```python
from build123d import *

# Parameters (mm, degrees)
F0_W     = 64.9276450276
F0_H     = 21.2974622846
F0_W_2   = 4.8806965351
F0_H_2   = 10.0571289659
F1_DEPTH = 25.4
F2_DEPTH = 25.4


with BuildPart() as f1:
    # F0 (on Right) → F1 (new body)
    with BuildSketch(Plane.YZ):
        Polygon((42.2991216183, -21.2974622846), (42.2991216183, 21.2974622846), (4.8806965351, 21.2974622846), (0, 21.2974622846), (-42.2991216183, 21.2974622846), (-42.2991216183, 0), (-42.2991216183, -21.2974622846), align=None)
        with Locations((-74.7629441321, 10.6487311423)):
            Rectangle(F0_W, F0_H)
        with Locations((2.4403482676, 26.3260267675)):
            Rectangle(F0_W_2, F0_H_2)
    extrude(amount=F1_DEPTH)

    # F2 (add): a face of the model
    f2_faces = [f1.faces().sort_by_distance(p)[0] for p in [
        (0, -20.5074649501, 3.1809669358),
    ]]
    extrude(f2_faces, amount=F2_DEPTH)


solid = f1.part
```
Here's how the part is built. I have some questions about the finished solid (model axes, mm). A direction names the side the tool comes from. Coordinates: 2 decimals unless noted, no trailing zeros. Order: outer loops, then holes, each group sorted by start corner. A loop starts at its lowest first (then second) coordinate and runs counter-clockwise, first axis right, second up.
1) Imagine slicing it at C-C on z = -17.5. List the corners of the cut face in (x, y) for me, and give its area (3 significant figures).
2) Will these pins go through, and if not, where does the flat tip stop? pin 1 (5 mm diameter, centred on x = 2.5, y = 23.5, fed in from +Z); pin 2 (17 mm diameter, centred on x = -8, z = -9.5, fed in from -Y); pin 3 (8 mm diameter, centred on x = -6.5, z = 28.5, fed in from +Y).
3) Which directions (+Z, -Z, +X, -X, +Y, -Y) give clear straight access to the entire face, cutting with the end or side of a thin tool? Please do faces 1 (the face through (0, -42.299, -10)), 2 (the face through (0, 24, 21.297)), 3 (the face through (0, 0, 26)).
4) Imagine slicing it at B-B on y = -57. List the corners of the cut face in (x, z) for me.
5) Imagine slicing it at A-A on x = -5. List the corners of the cut face in (y, z) for me.
6) I need wall thicknesses on line 1 (Y direction, x = 5.5, z = -5.5); line 2 (Z direction, x = 15, y = -81); line 3 (Y direction, x = 12.5, z = 29). Which ranges of each line are inside material? Lowest first, please.
Response values:
1. outline: (-25.4, -42.3) - (25.4, -42.3) - (25.4, 42.3) - (-25.4, 42.3) - close
1. area: 4,300 mm2
2. pin 1: stops at z = 21.3
2. pin 2: stops at y = -42.3
2. pin 3: stops at y = 4.88
3. face 1: -Z, +X, -X, -Y
3. face 2: +Z, +X, -X, +Y
3. face 3: +Z, +X, -X, -Y
4. outline: (-25.4, 0) - (25.4, 0) - (25.4, 21.3) - (-25.4, 21.3) - close
5. outline: (-107.23, 0) - (-42.3, 0) - (-42.3, -21.3) - (42.3, -21.3) - (42.3, 21.3) - (4.88, 21.3) - (4.88, 31.35) - (0, 31.35) - (0, 21.3) - (-107.23, 21.3) - close
6. line 1: y = -42.3 to 42.3
6. line 2: z = 0 to 21.3
6. line 3: y = 0 to 4.88
